Work out the finished part from the listing and answer in its coordinate system (mm). Face numbers are marked on the shaded views. Coordinates: 2 decimals unless noted, no trailing zeros. Write each loop counter-clockwise with the first axis right and the second up, starting at its lowest first coordinate (ties: lowest second). Pieces come first, ordered by that corner, then holes. Notation, with made-up numbers: (-13, 32) - (24, 32) arc R10 ccw to (24, 46) - close; hole circle Ø11 at (-17.75, -13.75). An arc over 180 degrees is marked (long way). One line per item, written item: value.
```python
from build123d import *

# Parameters (mm, degrees)
SKETCH1_R          = 56
EXTRUDE1_DEPTH     = 7.5
SKETCH2_R          = 10
EXTRUDE5_DEPTH     = 35
SKETCH5_R          = 45
EXTRUDE6_DEPTH     = 4
SKETCH6_R          = 4
EXTRUDE7_DEPTH     = 39.5
CHAMFER3_SIZE      = 1
EXTRUDE8_DEPTH     = 67
EXTRUDE10_DEPTH    = 67
SKETCH10_W         = 20
SKETCH10_H         = 12.483117272
EXTRUDE11_DEPTH    = 67
SKETCH11_R         = 7.5
EXTRUDE12_DEPTH    = 1.5
SKETCH12_R         = 10
EXTRUDE13_DEPTH    = 5
SKETCH13_R         = 7.5
EXTRUDE15_DEPTH    = 3
CHAMFER4_SIZE      = 1.5
CHAMFER6_SIZE      = 1.5
CHAMFER7_SIZE      = 1.5
SKETCH16_R         = 4
EXTRUDE16_DEPTH    = 10.5
SKETCH17_OUTSIDE_W = 146.672
SKETCH17_OUTSIDE_H = 146.672
SKETCH17_OUTSIDE_R = 51
EXTRUDE17_DEPTH    = 1.5
FILLET7_R          = 0.5


with BuildPart() as part:
    # Sketch1 → Extrude1 (new body)
    with BuildSketch(Plane(origin=(0, 0, 0), x_dir=(1, 0, 0), z_dir=(0, 1, 0))):
        with Locations(Location((0, 0, 0), (0, 0, 270))):  # turned: the seam where the file's is
            Circle(SKETCH1_R)
    extrude(amount=EXTRUDE1_DEPTH)

    # Sketch2 → Extrude5 (add)
    with BuildSketch(Plane.XZ):
        with Locations(Location((0, 0, 0), (0, 0, 90))):  # turned: the seam where the file's is
            Circle(SKETCH2_R)
    extrude(amount=EXTRUDE5_DEPTH)

    # Sketch5 → Extrude6 (cut)
    with BuildSketch(Plane(origin=(0, 7.5, 0), x_dir=(1, 0, 0), z_dir=(0, 1, 0))):
        with Locations(Location((0, 0, 0), (0, 0, 270))):  # turned: the seam where the file's is
            Circle(SKETCH5_R)
    extrude(amount=-EXTRUDE6_DEPTH, mode=Mode.SUBTRACT)

    # Sketch6 → Extrude7 (cut, through all)
    with BuildSketch(Plane(origin=(0, 3.5, 0), x_dir=(1, 0, 0), z_dir=(0, 1, 0))):
        with Locations(Location((0, 0, 0), (0, 0, 270))):  # turned: the seam where the file's is
            Circle(SKETCH6_R)
    extrude(amount=-EXTRUDE7_DEPTH, mode=Mode.SUBTRACT)

    # Chamfer3
    chamfer3_edges = [part.edges().sort_by_distance(p)[0] for p in [
        (0, 3.5, -4),
    ]]
    chamfer(chamfer3_edges, length=CHAMFER3_SIZE)

    # Sketch7 → Extrude8 (cut, through all)
    with BuildSketch(Plane.XY.offset(10)):
        Polygon((-10, -23), (-8.939339828, -23), (-8.939339828, -24.689339828), (-10, -25.75), align=None)
    extrude8 = extrude(amount=-EXTRUDE8_DEPTH, mode=Mode.SUBTRACT)

    # Mirror2: Extrude8 across plane
    add(extrude8.mirror(Plane(origin=(0, 0, 0), x_dir=(0, 0, 1), z_dir=(1, 0, 0))), mode=Mode.SUBTRACT)

    # Sketch9 → Extrude10 (cut, through all)
    with BuildSketch(Plane.XY.offset(10)):
        Polygon((-10, -35), (-10, -32.25), (-9.116116524, -33.133883476), (-9.116116524, -34.133883476), (-8.25, -35), align=None)
    extrude10 = extrude(amount=-EXTRUDE10_DEPTH, mode=Mode.SUBTRACT)

    # Mirror3: Extrude10 across plane
    add(extrude10.mirror(Plane(origin=(0, 0, 0), x_dir=(0, 0, 1), z_dir=(1, 0, 0))), mode=Mode.SUBTRACT)

    # Sketch10 → Extrude11 (cut, through all)
    with BuildSketch(Plane.XY.offset(10)):
        with Locations((0, -29.241558636)):
            Rectangle(SKETCH10_W, SKETCH10_H)
    extrude(amount=-EXTRUDE11_DEPTH, mode=Mode.SUBTRACT)

    # Sketch11 → Extrude12 (add)
    with BuildSketch(Plane.XZ.offset(23)):
        with Locations(Location((0, 0, 0), (0, 0, 270))):  # turned: the seam where the file's is
            Circle(SKETCH11_R)
    extrude(amount=EXTRUDE12_DEPTH)

    # Sketch12 → Extrude13 (add)
    with BuildSketch(Plane.XZ.offset(24.5)):
        with Locations(Location((0, 0, 0), (0, 0, 90))):  # turned: the seam where the file's is
            Circle(SKETCH12_R)
    extrude(amount=EXTRUDE13_DEPTH)

    # Sketch13 → Extrude15 (add)
    with BuildSketch(Plane.XZ.offset(29.5)):
        with Locations(Location((0, 0, 0), (0, 0, 270))):  # turned: the seam where the file's is
            Circle(SKETCH13_R)
    extrude(amount=EXTRUDE15_DEPTH)

    # Chamfer4
    chamfer4_edges = [part.edges().sort_by_distance(p)[0] for p in [
        (0, -32.5, 7.5),
    ]]
    chamfer(chamfer4_edges, length=CHAMFER4_SIZE)

    # Chamfer6
    chamfer6_edges = [part.edges().sort_by_distance(p)[0] for p in [
        (0, -24.5, -10),
    ]]
    chamfer(chamfer6_edges, length=CHAMFER6_SIZE)

    # Chamfer7
    chamfer7_edges = [part.edges().sort_by_distance(p)[0] for p in [
        (0, -29.5, -10),
    ]]
    chamfer(chamfer7_edges, length=CHAMFER7_SIZE)

    # Sketch16 → Extrude16 (cut, through all)
    with BuildSketch(Plane(origin=(0, -23, 0), x_dir=(-1, 0, 0), z_dir=(0, 1, 0))):
        with Locations(Location((0, 0, 0), (0, 0, 90))):  # turned: the seam where the file's is
            Circle(SKETCH16_R)
    extrude(amount=-EXTRUDE16_DEPTH, mode=Mode.SUBTRACT)

    # Sketch17 outside → Extrude17 (cut)
    with BuildSketch(Plane.XZ):
        Rectangle(SKETCH17_OUTSIDE_W, SKETCH17_OUTSIDE_H)
        with Locations(Location((0, 0, 0), (0, 0, 270))):  # turned: the seam where the file's is
            Circle(SKETCH17_OUTSIDE_R, mode=Mode.SUBTRACT)
    extrude(amount=-EXTRUDE17_DEPTH, mode=Mode.SUBTRACT)

    # Fillet7
    fillet7_edges = [part.edges().sort_by_distance(p)[0] for p in [
        (0, 3.5, -45),
    ]]
    fillet(fillet7_edges, radius=FILLET7_R)


solid = part.part
```
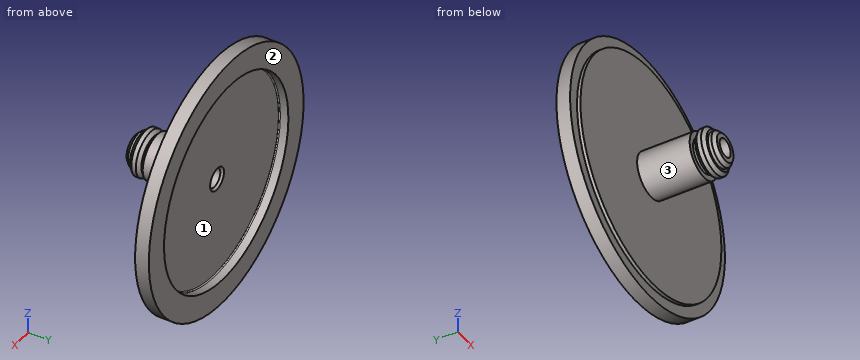
Item 1: Given pin 1 (1.5 mm diameter, centred on x = -29, z = -21.5, fed in from -Y); pin 2 (16 mm diameter, centred on x = 2, z = 0.5, fed in from -Y); pin 3 (6 mm diameter, centred on x = 21.5, z = 22, fed in from +Y); pin 4 (5 mm diameter, centred on x = -2, z = 0, fed in from +Y), each flat-ended and moving along its own axis, determine where each tip first touches the part or whether it passes through.
Evaluation:
pin 1: stops at y = 0
pin 2: stops at y = -32.5
pin 3: stops at y = 3.5
pin 4: stops at y = 3
Item 2: Section A-A, the plane y = -19 is taken. Determine the outline of the cut face in (x, z), then the cut area to 3 significant figures.
Evaluation:
outline: circle Ø20 at (0, 0); hole circle Ø8 at (0, 0)
area: 264 mm2
Item 3: Consider probe 1 along X at (y, z) = (4, 0); probe 2 along Y at (x, z) = (39.5, -25); probe 3 along Y at (x, z) = (-16.5, 37). Determine where each line is inside the solid, lowest interval first.
Evaluation:
probe 1: x = -56 to -45, 45 to 56
probe 2: y = 0 to 7.5
probe 3: y = 0 to 3.5
Item 4: Determine the mould class of the marked faces 1, 2 and 3 for opening direction Z: +Z half, -Z half, draft (parallel to the pull), parting line (faces both ways), or undercut.
Evaluation:
face 1: undercut
face 2: draft
face 3: parting line
